Autodesk Inventor part; units mm, degrees
ref_plane "YZ Plane" through (0, 0, 0) normal (1, 0, 0) x (0, 1, 0)
ref_plane "XZ Plane" through (0, 0, 0) normal (0, 1, 0) x (-1, 0, 0)
ref_plane "XY Plane" through (0, 0, 0) normal (0, 0, 1) x (1, 0, 0)
sketch "Sketch1" plane through (0, 0, 0) normal (0, 1, 0) x (-1, 0, 0)
  line L0 (0, 0) -> (515, 0) construction
  line L1 (515, 0) -> (515, -900)
  line L2 (515, -900) -> (0, -900) construction
  line L3 (0, -900) -> (0, 0)
  line L4 (500, 0) -> (465, 0) construction
  line L5 (465, 0) -> (465, 7.3489)
  line L6 (465, 7.3489) -> (500, 7.3489)
  line L7 (500, 7.3489) -> (500, 0)
  line L8 (275, 0) -> (240, 0) construction
  line L9 (240, 0) -> (240, 7.3489)
  line L10 (240, 7.3489) -> (275, 7.3489)
  line L11 (275, 7.3489) -> (275, 0)
  line L12 (515, 0) -> (500, 0)
  line L13 (0, 0) -> (240, 0) construction
  line L14 (465, 0) -> (275, 0)
  line L15 (0, -450) -> (515, -450) construction
  line L16 (465, -900) -> (465, -907.3489)
  line L17 (465, -907.3489) -> (500, -907.3489)
  line L18 (500, -907.3489) -> (500, -900)
  line L19 (240, -900) -> (240, -907.3489)
  line L20 (240, -907.3489) -> (275, -907.3489)
  line L21 (275, -907.3489) -> (275, -900)
  line L22 (0, -900) -> (240, -900) construction
  line L23 (275, -900) -> (465, -900)
  line L24 (500, -900) -> (515, -900)
  line L25 (50, 0) -> (15, 0) construction
  line L26 (15, 0) -> (15, 7.3489)
  line L27 (15, 7.3489) -> (50, 7.3489)
  line L28 (50, 7.3489) -> (50, 0)
  line L29 (240, 0) -> (50, 0)
  line L30 (15, 0) -> (0, 0)
  line L31 (50, -900) -> (15, -900) construction
  line L32 (15, -900) -> (15, -907.3489)
  line L33 (15, -907.3489) -> (50, -907.3489)
  line L34 (50, -907.3489) -> (50, -900)
  line L35 (240, -900) -> (50, -900)
  line L36 (15, -900) -> (0, -900)
  dimension "d0" = 900
  dimension "d1" = 515
  dimension "d4" = 35
  dimension "d5" = 35
  dimension "d6" = 190
  dimension "d7" = 15
  dimension "d8" = 240
  dimension "d9" = 190
extrude "Extrusion1" add sketch "Sketch1" along normal blind 6
properties part number "Superior_top" material "Wood (Oak)"
The listing builds one solid part. Answer for the finished solid, in the listing's coordinates (mm). Coordinates: 2 decimals unless noted, no trailing zeros. Write each loop counter-clockwise with the first axis right and the second up, starting at its lowest first coordinate (ties: lowest second). Pieces come first, ordered by that corner, then holes. Notation, with made-up numbers: (-20.75, 84.5) -> (34.25, 84.5) arc R22 cw to (34.25, 101.5) -> close; hole circle Ø9 at (86, -12). An arc over 180 degrees is marked (long way). Write each question's results on one line, items separated by ' | '. Start each with the question number.
1) A straight line is drawn through the part: probe 1 along Z at (x, y) = (-111.5, 2.7). Find the intervals that lie inside material, in ascending order.
2) Flat-ended cylindrical pins translate along their axes: pin 1 Ø1.8 at (x, y) = (-511, 4) entering from -Z; pin 2 Ø3 at (y, z) = (4, 2) entering from -X; pin 3 Ø3 at (x, y) = (-146, 2.5) entering from +Z. Find the tip coordinate at first contact, or state that the pin passes through.
3) A cutting plane is placed at A-A (x = -73). Determine the outline of the cut face in (y, z), then the cut area to 3 significant figures.
Values follow:
1) probe 1: -900 to 0
2) pin 1: z = -900 | pin 2: x = -500 | pin 3: z = 0
3) outline: (0, -900) -> (6, -900) -> (6, 0) -> (0, 0) -> close | area: 5,400 mm²
